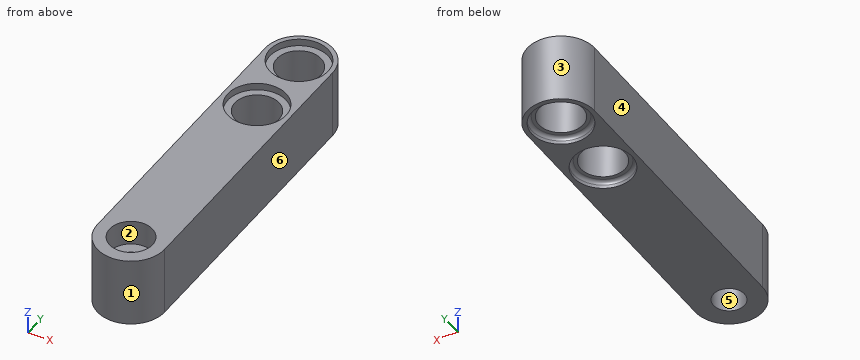
from build123d import *

# Parameters (mm, degrees)
F0_R      = 2.5
F1_DEPTH  = 7.8
F2_R      = 3.3
F3_DEPTH  = 0.8
F4_R      = 3.3
F5_DEPTH  = 0.8
F6_R      = 2.425
F7_DEPTH  = 2.8
F8_R      = 1.75
F9_DEPTH  = 4
F10_R     = 1.15
F11_DEPTH = 5.001
F12_R     = 0.59999
F13_R     = 0.4


# Not quite as in the source:
# - a fillet or chamfer is up to 0.001 mm smaller than in the source, because OpenCascade refuses the exact size


with BuildPart() as f1:
    # F0 (on Top) → F1 (new body)
    with BuildSketch(Plane.XY):
        with BuildLine():
            Line((0, 32), (0, 0))
            ThreePointArc((0, 0), (3.8, -3.8), (7.6, 0))
            Line((7.6, 0), (7.6, 32))
            ThreePointArc((7.6, 32), (3.8, 35.8), (0, 32))
        make_face()
        with Locations((3.8, 24)):
            Circle(F0_R, mode=Mode.SUBTRACT)
        with Locations((3.8, 32)):
            Circle(F0_R, mode=Mode.SUBTRACT)
    extrude(amount=F1_DEPTH)

    # F2 (on face) → F3 (cut)
    with BuildSketch(Plane.XY.offset(7.8)):
        with Locations((3.8, 32)):
            Circle(F2_R)
        with Locations((3.8, 24)):
            Circle(F2_R)
    extrude(amount=-F3_DEPTH, mode=Mode.SUBTRACT)

    # F4 (on face) → F5 (cut)
    with BuildSketch(Plane(origin=(0, 0, 0), x_dir=(1, 0, 0), z_dir=(0, 0, -1))):
        with Locations((3.8, -24)):
            Circle(F4_R)
        with Locations((3.8, -32)):
            Circle(F4_R)
    extrude(amount=-F5_DEPTH, mode=Mode.SUBTRACT)

    # F6 (on face) → F7 (cut)
    with BuildSketch(Plane.XY.offset(7.8)):
        with Locations((3.8, 0)):
            Circle(F6_R)
    extrude(amount=-F7_DEPTH, mode=Mode.SUBTRACT)

    # F8 (on face) → F9 (cut)
    with BuildSketch(Plane(origin=(0, 0, 0), x_dir=(1, 0, 0), z_dir=(0, 0, -1))):
        with Locations((3.8, 0)):
            Circle(F8_R)
    extrude(amount=-F9_DEPTH, mode=Mode.SUBTRACT)

    # F10 (on face) → F11 (cut, through all)
    with BuildSketch(Plane.XY.offset(5)):
        with Locations((3.8, 0)):
            Circle(F10_R)
    extrude(amount=-F11_DEPTH, mode=Mode.SUBTRACT)

    # F12 (radius 0.6 in the source; OpenCascade refuses exactly that, so slightly less here)
    f12_edges = [f1.edges().sort_by_distance(p)[0] for p in [
        (2.05, 0, 4),
    ]]
    fillet(f12_edges, radius=F12_R)

    # F13
    f13_edges = [f1.edges().sort_by_distance(p)[0] for p in [
        (0.5, 24, 0.8),
        (0.5, 32, 0.8),
    ]]
    fillet(f13_edges, radius=F13_R)


solid = f1.part
CAD build for the part. Positions are in the model's coordinates, mm. Face numbers are marked on the shaded views. A direction names the side the tool comes from. Round coordinates to 2 decimals unless told otherwise and drop trailing zeros. Write each loop counter-clockwise with the first axis right and the second up, starting at its lowest first coordinate (ties: lowest second). Pieces come first, ordered by that corner, then holes.
(1) Drop flat-ended pins along their axis: P1, Ø1.8, axis at x = 3.5, y = -0.5, coming from the -Z side; P2, Ø4, axis at x = 3.8, y = 0, coming from the +Z side. Give the stop position or say it passes through.
(2) 3-axis set-ups, long thin cutter, end or side, ignore diameter. For the marked faces 5 and 6: which of +Z, -Z, +X, -X, +Y, -Y reach the whole face in a straight line?
(3) Slice it at C-C, the plane x = 3.8. Count the separate pieces of the cut face and the enclosed holes in it, and give its area (3 significant figures).
(4) Mould opens along Y. For the marked faces 1, 2, 3 and 4 say: pulls with the +Y half, pulls with the -Y half, needs draft (parallel to the pull), parting line crosses it, or undercut.
(5) Probe line 1 along Y through (x, z) = (3.8, 0.9); line 2 along Y through (x, z) = (3.8, 7.55) (3 decimals); line 3 along X through (y, z) = (24, 0.1). List the from-to ranges inside material, lowest first.
(6) Slice it at A-A, the plane y = 24. Write the cut outline in (x, z).
(7) Slice it at B-B, the plane z = 1.75. Write the cut outline in (x, y).
From the geometry:
1. P1: stops at z = 3.9
1. P2: stops at z = 5
2. face 5: -Z
2. face 6: +Z, -Z, +X, +Y, -Y
3. separate pieces: 4
3. enclosed holes: 0
3. area: 196 mm2
4. face 1: pulls with the -Y half
4. face 2: undercut
4. face 3: pulls with the +Y half
4. face 4: needs draft
5. line 1: y = -3.8 to -1.75, 1.75 to 21.5, 26.5 to 29.5, 34.5 to 35.8
5. line 2: y = -3.8 to -2.425, 2.425 to 20.7, 27.3 to 28.7, 35.3 to 35.8
5. line 3: x = 0 to 0.5, 7.1 to 7.6
6. outline: (0, 0) - (0.5, 0) - (0.5, 0.4) arc R0.4 cw to (0.9, 0.8) - (1.3, 0.8) - (1.3, 7) - (0.5, 7) - (0.5, 7.8) - (0, 7.8) - close; (6.3, 0.8) - (6.7, 0.8) arc R0.4 cw to (7.1, 0.4) - (7.1, 0) - (7.6, 0) - (7.6, 7.8) - (7.1, 7.8) - (7.1, 7) - (6.3, 7) - close
7. outline: (0, 0) arc R3.8 ccw to (7.6, 0) - (7.6, 32) arc R3.8 ccw to (0, 32) - close; hole circle Ø5 at (3.8, 24); hole circle Ø5 at (3.8, 32); hole circle Ø3.5 at (3.8, 0)
